from build123d import *

# Parameters (mm, degrees)
PAD013_DEPTH    = 5
SKETCH019_W     = 8
SKETCH019_H     = 5
POCKET001_DEPTH = 10
SKETCH020_W     = 3.1
SKETCH020_H     = 5
POCKET002_DEPTH = 10


with BuildPart() as part:
    # Sketch018 → Pad013 (new body)
    with BuildSketch(Plane.XY):
        with BuildLine():
            Line((-43.25, 0), (41.45, 0))
            ThreePointArc((41.45, 0), (42.722792, 0.527208), (43.25, 1.8))
            Line((43.25, 1.8), (43.25, 5.5))
            Line((43.25, 5.5), (21.25, 5.5))
            Line((21.25, 5.5), (21.25, 2.65))
            Line((21.25, 2.65), (17.75, 2.65))
            Line((17.75, 2.65), (17.75, 5.5))
            Line((-14.75, 5.5), (17.75, 5.5))
            Line((-14.75, 2.65), (-14.75, 5.5))
            Line((-18.25, 2.65), (-14.75, 2.65))
            Line((-18.25, 5.5), (-18.25, 2.65))
            Line((-43.25, 5.5), (-18.25, 5.5))
            Line((-43.25, 5.5), (-43.25, 0))
        make_face()
    extrude(amount=PAD013_DEPTH)

    # Sketch019 → Pocket001 (cut)
    with BuildSketch(Plane.XZ):
        with Locations((11.25, -0.5)):
            Rectangle(SKETCH019_W, SKETCH019_H)
    extrude(amount=-POCKET001_DEPTH, mode=Mode.SUBTRACT)

    # Sketch020 → Pocket002 (cut)
    with BuildSketch(Plane.XZ):
        with Locations((-29.8, 0.5)):
            Rectangle(SKETCH020_W, SKETCH020_H)
    extrude(amount=-POCKET002_DEPTH, mode=Mode.SUBTRACT)


with BuildPart() as part_1:
    # Body010 placement: moved
    add(part.part.moved(Location((0, 0, -102))))


solid = part_1.part
Input: part model. Units: mm. Frame: model coordinates. A direction names the side the tool comes from. Give positions to 0.01 mm unless a question says otherwise; leave off trailing zeros. Write each loop counter-clockwise with the first axis right and the second up, starting at its lowest first coordinate (ties: lowest second). Pieces come first, ordered by that corner, then holes. Notation, with made-up numbers: (67, -34.5) -> (124, -34.5) arc R19 ccw to (124, -28.5) -> close; hole circle Ø5 at (-9, 20). An arc over 180 degrees is marked (long way). Use one line per item in the form item = value. Start each with the question number.
1) Section query B-B on x = -17. Return the cut outline in (y, z), then the cut area to 4 significant figures.
2) Pin query (flat end, axial travel): pin 1 (0.9 mm diameter, centred on x = -29.5, y = 1.5, fed in from -Z); pin 2 (3 mm diameter, centred on x = 19.5, z = -98.5, fed in from +Y). Return the tip coordinate at first contact, or that it passes through.
3) Section query A-A on y = 3.35. Return the cut outline in (x, z), then the cut area to 3 significant figures.
4) Ray query, probe 1 along X at (y, z) = (2.25, -100.1); probe 2 along X at (y, z) = (3.85, -97.4); probe 3 along X at (y, z) = (4.65, -99.65). Return the intervals inside material, ascending. Write a range as from..to.
5) Set-up query: faces 1 (the flat face through (-1, 0, -100)), 2 (the flat face through (-18.25, 4, -100)), 3 (the flat face through (15.25, 3, -101)). Return all of +Z, -Z, +X, -X, +Y, -Y with unobstructed straight access to the full face (end or side cutting, diameter ignored); none if empty.
6) Draft query along X for faces 4 (the flat face through (21.25, 4, -100)), 5 (the flat face through (1, 5.5, -100)), 6 (the flat face through (-43.25, 3, -100)). Return one class per face: pulls with the +X half, pulls with the -X half, needs draft (parallel to the pull), parting line crosses it, or undercut.
7) Section query C-C on x = 14.5. Return the cut outline in (y, z), then the cut area to 3 significant figures.
Outcome:
q1.outline = (0, -102) -> (2.65, -102) -> (2.65, -97) -> (0, -97) -> close
q1.area = 13.25 mm^2
q2.pin_1 = -99
q2.pin_2 = 2.65
q3.outline = (-43.25, -102) -> (-31.35, -102) -> (-31.35, -99) -> (-28.25, -99) -> (-28.25, -102) -> (-18.25, -102) -> (-18.25, -97) -> (-43.25, -97) -> close; (-14.75, -102) -> (7.25, -102) -> (7.25, -100) -> (15.25, -100) -> (15.25, -102) -> (17.75, -102) -> (17.75, -97) -> (-14.75, -97) -> close; (21.25, -102) -> (43.25, -102) -> (43.25, -97) -> (21.25, -97) -> close
q3.area = 372 mm^2
q4.probe_1 = -43.25..-31.35, -28.25..7.25, 15.25..43.25
q4.probe_2 = -43.25..-18.25, -14.75..17.75, 21.25..43.25
q4.probe_3 = -43.25..-31.35, -28.25..-18.25, -14.75..17.75, 21.25..43.25
q5.face_1 = +Z, -Z, +X, -X, -Y
q5.face_2 = +Z, -Z, +Y
q5.face_3 = -Z, +Y, -Y
q6.face_4 = undercut
q6.face_5 = needs draft
q6.face_6 = pulls with the -X half
q7.outline = (0, -100) -> (5.5, -100) -> (5.5, -97) -> (0, -97) -> close
q7.area = 16.5 mm^2
